Source: three-view drawing plus pictorial views. Frame: mm from the lowest corner of the part. Give positions to 0.01 mm unless a question says otherwise; leave off trailing zeros. Write each loop counter-clockwise with the first axis right and the second up, starting at its lowest first coordinate (ties: lowest second). Pieces come first, ordered by that corner, then holes. Notation, with made-up numbers: (47.25, -13.5) -> (85.25, -13.5) arc R36 cw to (85.25, 23.5) -> close; hole circle Ø11 at (15, -27.5). An arc over 180 degrees is marked (long way). Use a Markdown table: item, result. Add a question column.
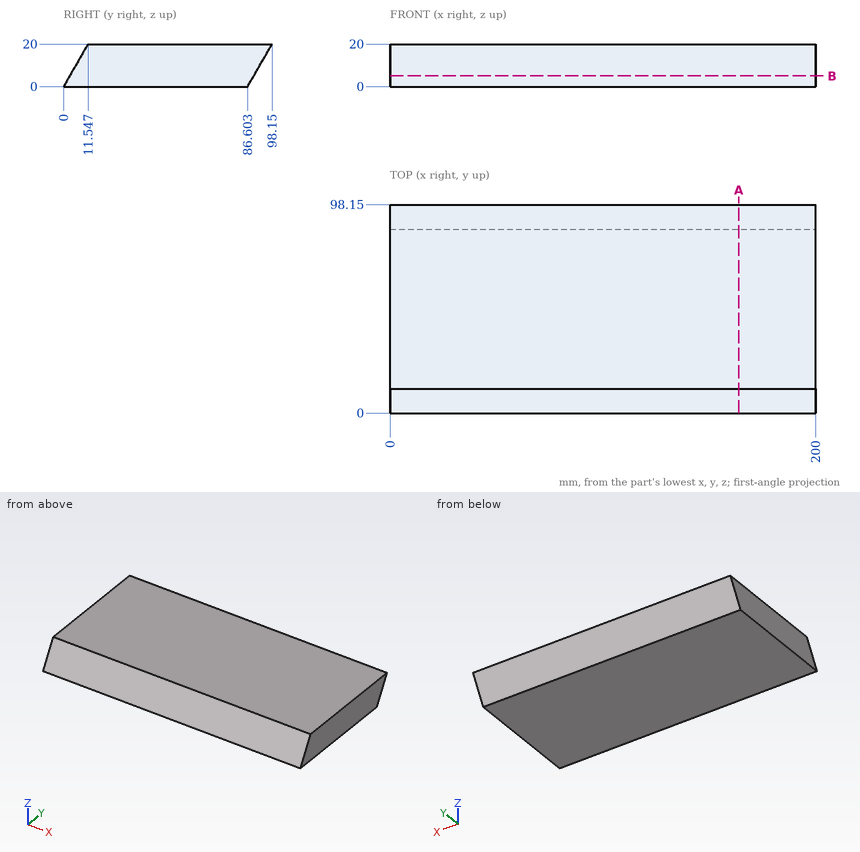
(1) First-contact query: pin 1 Ø10 at (x, z) = (129, 9) entering from +Y; pin 2 Ø10 at (x, z) = (48, 7) entering from -Y; pin 3 Ø6 at (y, z) = (34, 7.5) entering from -X; pin 4 Ø5 at (x, z) = (97.5, 6) entering from +Y. Flat tips, straight axial feed; report the tip coordinate or a pass-through.
(2) Material intervals for L1, parallel to Y at x = 54, z = 9.5; L2, parallel to Y at x = 115, z = 4; L3, parallel to Z at x = 26.5, y = 9, sorted ascending.
(3) Cut plane A-A on x = 164. Return the cut outline in (y, z).
(4) Cut plane B-B on z = 5. Return the cut outline in (x, y).
Output:
| question | item | result |
|---|---|---|
| 1 | pin 1 | y = 94.69 |
| 1 | pin 2 | y = 1.15 |
| 1 | pin 3 | x = 0 |
| 1 | pin 4 | y = 91.51 |
| 2 | L1 | 5.48 to 92.09 |
| 2 | L2 | 2.31 to 88.91 |
| 2 | L3 | 0 to 15.59 |
| 3 | outline | (0, 0) -> (86.6, 0) -> (98.15, 20) -> (11.55, 20) -> close |
| 4 | outline | (0, 2.89) -> (200, 2.89) -> (200, 89.49) -> (0, 89.49) -> close |
